The listing builds one solid part. Answer for the finished solid, in the listing's coordinates (mm). Face numbers are marked on the shaded views. A direction names the side the tool comes from. Give positions to 0.01 mm unless a question says otherwise; leave off trailing zeros. Loops run counter-clockwise (first coordinate to the right, second up) from the corner with the lowest first, then second, coordinate; pieces in that order, holes last.
Item 1: Each of these flat-tipped pins is pushed along its axis until it touches: pin 1 Ø0.8 at (y, z) = (0.5, 60.5) entering from +X (3 decimals); pin 2 Ø3 at (y, z) = (14.29, 82.55) entering from +X; pin 3 Ø12 at (x, z) = (19, 71.5) entering from +Y; pin 4 Ø10 at (x, z) = (2.5, 133) entering from -Y. Where does it stop, or does it pass through?
Item 2: Section C-C, the plane y = 6.35 is taken. Give the vertices of the cut face in (x, z).
Item 3: Consider line 1 along Y through (x, z) = (1.05, 19.05); line 2 along Y through (x, z) = (1.25, 165.1); line 3 along X through (y, z) = (19.75, 102). Determine where each line is inside the solid, lowest interval first.
Item 4: Section B-B, the plane z = 19.05 is taken. Give the vertices of the cut face in (x, y), and give its area (3 significant figures).
Item 5: A tool of negligible diameter and unlimited length cuts with its end or side. For the marked faces 1 and 2, from which of +Z, -Z, +X, -X, +Y, -Y can it reach the whole face along a straight path? Write none if from no direction.
Item 6: Section D-D, the plane z = 104.5 is taken. Give the vertices of the cut face in (x, y).
Item 7: Section A-A, the plane x = 12.25 is taken. Give the vertices of the cut face in (y, z).
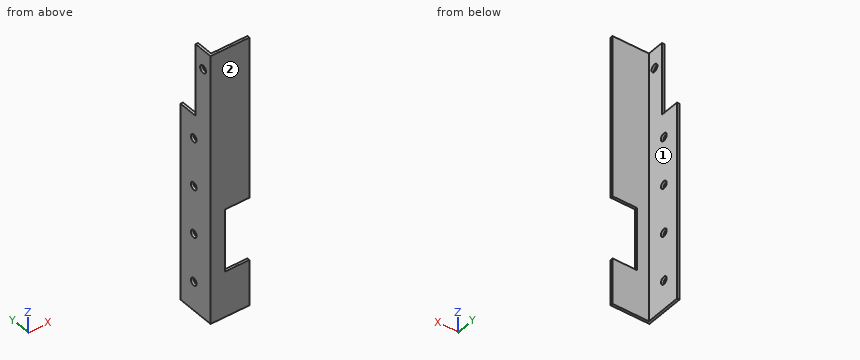
from build123d import *

# Parameters (mm, degrees)
BOSS_EXTRUDE1_DEPTH          = 177.8
F_10_0_1935_DIAMETER_HOLE1_D = 4.9149
SKETCH4_W                    = 15.875
SKETCH4_H                    = 41.275
CUT_EXTRUDE1_DEPTH           = 2.6002
SKETCH5_W                    = 47.625
SKETCH5_H                    = 12.7
CUT_EXTRUDE2_DEPTH           = 2.6002
F_10_0_1935_DIAMETER_HOLE2_D = 4.9149


with BuildPart() as part:
    # Sketch1 → Boss-Extrude1 (new body)
    with BuildSketch(Plane.XY):
        Polygon((0, 0), (0, 25.4), (1.6002, 25.4), (1.6002, 1.6002), (25.4, 1.6002), (25.4, 0), align=None)
    extrude(amount=BOSS_EXTRUDE1_DEPTH)

    # #10 (0.1935) Diameter Hole1 (through all)
    with Locations(Plane(origin=(1.6002, 0, 0), x_dir=(0, 0, -1), z_dir=(1, 0, 0))):
        with Locations((-82.55, 14.2875), (-50.8, 14.2875), (-19.05, 14.2875), (-114.3, 14.2875)):
            Hole(F_10_0_1935_DIAMETER_HOLE1_D / 2)

    # Sketch4 → Cut-Extrude1 (cut, through all)
    with BuildSketch(Plane(origin=(0, 1.6002, 0), x_dir=(1, 0, 0), z_dir=(0, 1, 0))):
        with Locations((17.4625, -50.8)):
            Rectangle(SKETCH4_W, SKETCH4_H)
    extrude(amount=-CUT_EXTRUDE1_DEPTH, mode=Mode.SUBTRACT)

    # Sketch5 → Cut-Extrude2 (cut, through all)
    with BuildSketch(Plane(origin=(1.6002, 0, 0), x_dir=(0, 0, -1), z_dir=(1, 0, 0))):
        with Locations((-153.9875, 19.05)):
            Rectangle(SKETCH5_W, SKETCH5_H)
    extrude(amount=-CUT_EXTRUDE2_DEPTH, mode=Mode.SUBTRACT)

    # #10 (0.1935) Diameter Hole2 (through all)
    with Locations(Plane(origin=(1.6002, 0, 0), x_dir=(0, 0, -1), z_dir=(1, 0, 0))):
        with Locations((-165.1, 6.35)):
            Hole(F_10_0_1935_DIAMETER_HOLE2_D / 2)


solid = part.part
Worked answers:
1. pin 1: stops at x = 9.525
1. pin 2: passes through
1. pin 3: stops at y = 1.6
1. pin 4: stops at y = 0
2. outline: (0, 0) - (1.6, 0) - (1.6, 162.64) - (0, 162.64) - close; (0, 167.56) - (1.6, 167.56) - (1.6, 177.8) - (0, 177.8) - close
3. line 1: y = 0 to 11.83, 16.74 to 25.4
3. line 2: y = 0 to 3.89, 8.81 to 12.7
3. line 3: x = 0 to 1.6
4. outline: (0, 0) - (25.4, 0) - (25.4, 1.6) - (1.6, 1.6) - (1.6, 11.83) - (0, 11.83) - close; (0, 16.74) - (1.6, 16.74) - (1.6, 25.4) - (0, 25.4) - close
4. area: 70.9 mm2
5. face 1: +Z, -Z, +X, +Y
5. face 2: +Z, -Z, +X, -X, -Y
6. outline: (0, 0) - (25.4, 0) - (25.4, 1.6) - (1.6, 1.6) - (1.6, 25.4) - (0, 25.4) - close
7. outline: (0, 0) - (1.6, 0) - (1.6, 30.16) - (0, 30.16) - close; (0, 71.44) - (1.6, 71.44) - (1.6, 177.8) - (0, 177.8) - close
